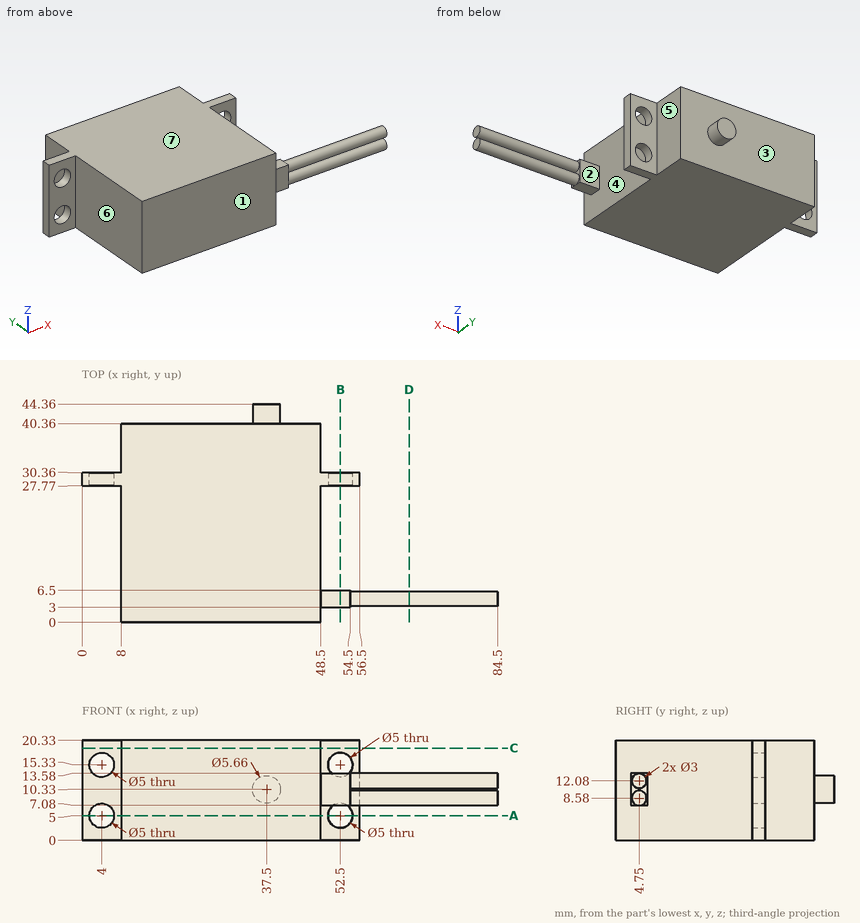
Here's the drawing with two shaded views (mm, measured from the low corner). I have some questions. A direction names the side the tool comes from. Give positions to 0.01 mm unless a question says otherwise; leave off trailing zeros. Loops run counter-clockwise (first coordinate to the right, second up) from the corner with the lowest first, then second, coordinate; pieces in that order, holes last. Notation, with made-up numbers: M 13.5,61.5 L 39.5,61.5 A11 ccw 39.5,67.5 Z; hole C -18.5,24 d9. An arc over 180 degrees is marked long. Answer in a Markdown table with one row per item.
1. For pin 1 Ø3 at (y, z) = (30, 18) entering from +X; pin 2 Ø4 at (x, z) = (53.5, 5.5) entering from +Y; pin 3 Ø8 at (y, z) = (12.5, 9.5) entering from +X; pin 4 Ø1 at (x, z) = (61.5, 14.5) entering from -Y, each with a flat end and sliding along its axis, tell me the tip position at first contact or that it passes through.
Taken from the geometry:
| item | result |
|---|---|
| pin 1 | stops at x = 56.5 |
| pin 2 | stops at y = 30.36 |
| pin 3 | stops at x = 48.5 |
| pin 4 | passes through |
2. Thinking about a two-plate mould opening in Y: for the marked faces 1, 2, 3 and 4, which applies, released by +Y, released by -Y, zero draft, split by the parting line, or undercut?
Taken from the geometry:
| item | result |
|---|---|
| face 1 | released by -Y |
| face 2 | undercut |
| face 3 | released by +Y |
| face 4 | undercut |
3. Suppose I cut it at A-A on z = 5. Write out the boundary of the cut face in (x, y).
Taken from the geometry:
| item | result |
|---|---|
| outline | M 0,27.77 L 1.5,27.77 L 1.5,30.36 L 0,30.36 Z; M 6.5,27.77 L 8,27.77 L 8,0 L 48.5,0 L 48.5,27.77 L 50,27.77 L 50,30.36 L 48.5,30.36 L 48.5,40.36 L 8,40.36 L 8,30.36 L 6.5,30.36 Z; M 55,27.77 L 56.5,27.77 L 56.5,30.36 L 55,30.36 Z |
4. Suppose I cut it at B-B on x = 52.5. Write out the boundary of the cut face in (y, z).
Taken from the geometry:
| item | result |
|---|---|
| outline | M 3,7.08 L 6.5,7.08 L 6.5,13.58 L 3,13.58 Z; M 27.77,0 L 30.36,0 L 30.36,2.5 L 27.77,2.5 Z; M 27.77,7.5 L 30.36,7.5 L 30.36,12.83 L 27.77,12.83 Z; M 27.77,17.83 L 30.36,17.83 L 30.36,20.33 L 27.77,20.33 Z |
5. Suppose I cut it at C-C on z = 18.75. Write out the boundary of the cut face in (x, y).
Taken from the geometry:
| item | result |
|---|---|
| outline | M 0,27.77 L 8,27.77 L 8,0 L 48.5,0 L 48.5,27.77 L 56.5,27.77 L 56.5,30.36 L 48.5,30.36 L 48.5,40.36 L 8,40.36 L 8,30.36 L 0,30.36 Z |
6. Which directions (+Z, -Z, +X, -X, +Y, -Y) give clear straight access to the entire face, cutting with the end or side of a thin tool? Please do the marked faces 5, 6 and 7.
Taken from the geometry:
| item | result |
|---|---|
| face 5 | +Z, -Z, +X, +Y |
| face 6 | +Z, -Z, -X, -Y |
| face 7 | +Z, +X, -X, +Y, -Y |
7. Suppose I cut it at D-D on x = 66.5. Write out the boundary of the cut face in (y, z).
Taken from the geometry:
| item | result |
|---|---|
| outline | C 4.75,8.58 d3; C 4.75,12.08 d3 |
8. If I drill on line 1 along X through (y, z) = (28.6, 15.33); line 2 along Z through (x, y) = (4, 28.9); line 3 along Z through (x, y) = (52, 29), over which ranges is the centre line in solid material (lowest first)?
Taken from the geometry:
| item | result |
|---|---|
| line 1 | x = 0 to 1.5, 6.5 to 50, 55 to 56.5 |
| line 2 | z = 0 to 2.5, 7.5 to 12.83, 17.83 to 20.33 |
| line 3 | z = 0 to 2.55, 7.45 to 12.88, 17.78 to 20.33 |
